Autodesk Inventor part; units mm, degrees
ref_plane "YZ Plane" through (0, 0, 0) normal (1, 0, 0) x (0, 1, 0)
ref_plane "XZ Plane" through (0, 0, 0) normal (0, 1, 0) x (-1, 0, 0)
ref_plane "XY Plane" through (0, 0, 0) normal (0, 0, 1) x (1, 0, 0)
sketch "スケッチ1" plane through (0, 0, 0) normal (0, 1, 0) x (-1, 0, 0)
  circle A0 centre (0, 0) radius 17.5
  line L0 (8.124, 15.5) -> (8.124, -15.5)
  line L1 (-8.124, 15.5) -> (-8.124, -15.5)
  line L2 (4.6, 10.5) -> (-4.6, 10.5)
  line L3 (-4.6, 10.5) -> (-4.6, -10.5)
  line L4 (-4.6, -10.5) -> (4.6, -10.5)
  line L5 (4.6, -10.5) -> (4.6, 10.5)
  point P0 (4.6, 0)
  point P1 (0, 10.5)
  dimension "d0" = 35
  dimension "d1" = 31
  dimension "d2" = 9.2
  dimension "d3" = 21
extrude "押し出し1" add sketch "スケッチ1" along normal blind 1.2 contours L0 A0 L1
properties part number "ServoMotor_Holder"
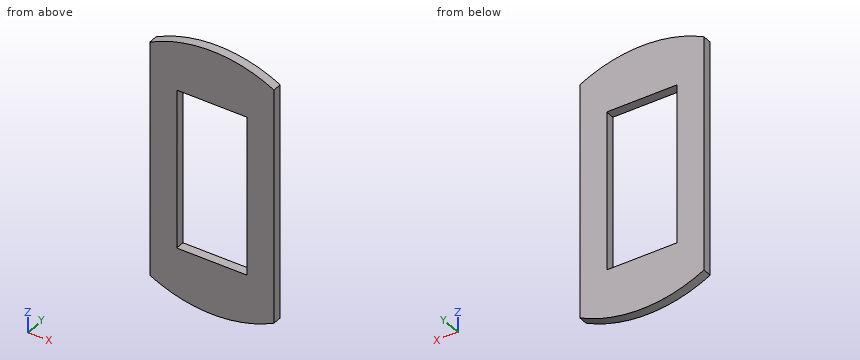
Geometry: final body of the model. Coordinates: model frame, mm. Coordinates: 2 decimals unless noted, no trailing zeros. Order: outer loops, then holes, each group sorted by start corner. A loop starts at its lowest first (then second) coordinate and runs counter-clockwise, first axis right, second up. Notation, with made-up numbers: (-36.5, 13.5) - (-13.5, 13.5) arc R15 cw to (-13.5, 18.5) - close; hole circle Ø2 at (18.5, 52.5). An arc over 180 degrees is marked (long way). Write each question's results on one line, items separated by ' | '.
1) Section D-D, the plane x = -5. Return loops of the section in (y, z), plus the area to 3 significant figures.
Results list:
outline: (0, -16.77) - (1.2, -16.77) - (1.2, 16.77) - (0, 16.77) - close | area: 40.2 mm^2
2) Line query: line 1 (X direction, y = 0.2, z = 5); line 2 (Z direction, x = -3, y = 1); line 3 (Z direction, x = -2.5, y = 0.85). Output: solid intervals per line, ascending. Write a range as from..to.
Results list:
line 1: -8.12..-4.6, 4.6..8.12 | line 2: -17.24..-10.5, 10.5..17.24 | line 3: -17.32..-10.5, 10.5..17.32
3) Section B-B, the plane z = 4. Return loops of the section in (x, y), plus the area to 3 significant figures.
Results list:
outline: (-8.12, 0) - (-4.6, 0) - (-4.6, 1.2) - (-8.12, 1.2) - close; (4.6, 0) - (8.12, 0) - (8.12, 1.2) - (4.6, 1.2) - close | area: 8.46 mm^2
4) Section C-C, the plane y = 0.6. Return loops of the section in (x, z).
Results list:
outline: (-8.12, -15.5) arc R17.5 ccw to (8.12, -15.5) - (8.12, 15.5) arc R17.5 ccw to (-8.12, 15.5) - close; hole (-4.6, -10.5) - (4.6, -10.5) - (4.6, 10.5) - (-4.6, 10.5) - close
5) Section A-A, the plane x = 0. Return loops of the section in (y, z).
Results list:
outline: (0, -17.5) - (1.2, -17.5) - (1.2, -10.5) - (0, -10.5) - close; (0, 10.5) - (1.2, 10.5) - (1.2, 17.5) - (0, 17.5) - close
